Model file for the job. Use its own axes, mm. A direction names the side the tool comes from. Round coordinates to 2 decimals unless told otherwise and drop trailing zeros. Use a Markdown table: item, result. Add a question column.
Item 1: Tool access for faces 1 (the flat face through (-1, -304.8, 3)), 2 (the cylindrical face through (-219.67, -4.27, -106.67)): list every direction of +Z, -Z, +X, -X, +Y, -Y with a clear straight run to the whole face (end or side of a thin tool).
Item 2: Saw through at A-A on y = -169. Give the number of separate pieces and of enclosed holes in the cut face, then the cut area to 3 significant figures.
Item 3: Wall check: L1, parallel to X at y = -106, z = 20; L2, parallel to X at y = -13, z = -317; L3, parallel to X at y = 91, z = 204. Give the ranges that are in metal, low to high. Write a range as from..to.
Item 4: Two-plate mould, pull along X, no slides. Class faces 3 (the flat face through (3, -4, -228.6)), 4 (the cylindrical face through (-243.23, -4.09, 8.38)), 5 (the cylindrical face through (243.23, -4.09, -8.38)), 6 (the flat face through (4, -4, 584.2)): +X half, -X half, draft (parallel to the pull), parting line (faces both ways), or undercut.
Item 5: Pin check, flat tips, straight feed: P1, Ø10, axis at y = -227, z = -224, coming from the -X side; P2, Ø2, axis at y = -164.5, z = -183, coming from the -X side; P3, Ø1, axis at y = 111, z = -388.5, coming from the -X side. Stop position of each tip, or through.
```python
from build123d import *

# Parameters (mm, degrees)
F1_DEPTH = 304.8
F2_R     = 12.7
F4_DEPTH = 609.601


with BuildPart() as f1:
    # F0 (on Front) → F1 (new body, symmetric)
    with BuildSketch(Plane.XZ):
        with BuildLine():
            Line((304.8, 609.6), (-304.8, 609.6))
            ThreePointArc((-304.8, 609.6), (-243.217894, 0), (-304.8, -609.6))
            Line((-304.8, -609.6), (304.8, -609.6))
            ThreePointArc((304.8, -609.6), (243.217894, 0), (304.8, 609.6))
        make_face()
    extrude(amount=F1_DEPTH, both=True)

    # F2
    f2_edges = [f1.edges().sort_by_distance(p)[0] for p in [
        (304.8, 0, 609.6),
        (0, -304.8, 609.6),
        (-304.8, 0, 609.6),
        (0, 304.8, 609.6),
        (0, -304.8, -609.6),
        (304.8, 0, -609.6),
        (0, 304.8, -609.6),
        (-304.8, 0, -609.6),
        (243.217894, -304.8, 0),
        (-243.217894, -304.8, 0),
        (243.217894, 304.8, 0),
        (-243.217894, 304.8, 0),
    ]]
    fillet(f2_edges, radius=F2_R)

    # F3 (on face) → F4 (cut, through all)
    with BuildSketch(Plane.XZ.offset(304.8)):
        with BuildLine():
            ThreePointArc((248.302135, 431.8), (260.119024, 508.160601), (273.851838, 584.2))
            Line((273.851838, 584.2), (-273.851838, 584.2))
            ThreePointArc((-273.851838, 584.2), (-260.119024, 508.160601), (-248.302135, 431.8))
            Line((-248.302135, 431.8), (248.302135, 431.8))
        make_face()
        with BuildLine():
            ThreePointArc((273.851838, -584.2), (260.119024, -508.160601), (248.302135, -431.8))
            Line((248.302135, -431.8), (-248.302135, -431.8))
            ThreePointArc((-248.302135, -431.8), (-260.119024, -508.160601), (-273.851838, -584.2))
            Line((-273.851838, -584.2), (273.851838, -584.2))
        make_face()
        with BuildLine():
            ThreePointArc((244.805808, -406.4), (234.275634, -317.634344), (226.331339, -228.6))
            Line((226.331339, -228.6), (-226.331339, -228.6))
            ThreePointArc((-226.331339, -228.6), (-234.275634, -317.634344), (-244.805808, -406.4))
            Line((-244.805808, -406.4), (244.805808, -406.4))
        make_face()
        with BuildLine():
            ThreePointArc((224.542607, -203.2), (219.716122, -108.001944), (217.844134, -12.7))
            Line((217.844134, -12.7), (-217.844134, -12.7))
            ThreePointArc((-217.844134, -12.7), (-219.716122, -108.001944), (-224.542607, -203.2))
            Line((-224.542607, -203.2), (224.542607, -203.2))
        make_face()
        with BuildLine():
            ThreePointArc((217.844134, 12.7), (219.716122, 108.001944), (224.542607, 203.2))
            Line((224.542607, 203.2), (-224.542607, 203.2))
            ThreePointArc((-224.542607, 203.2), (-219.716122, 108.001944), (-217.844134, 12.7))
            Line((-217.844134, 12.7), (217.844134, 12.7))
        make_face()
        with BuildLine():
            ThreePointArc((226.331339, 228.6), (234.275634, 317.634344), (244.805808, 406.4))
            Line((244.805808, 406.4), (-244.805808, 406.4))
            ThreePointArc((-244.805808, 406.4), (-234.275634, 317.634344), (-226.331339, 228.6))
            Line((-226.331339, 228.6), (226.331339, 228.6))
        make_face()
    extrude(amount=-F4_DEPTH, mode=Mode.SUBTRACT)


solid = f1.part
```
Entries:
| question | item | result |
|---|---|---|
| 1 | face 1 | +Z, -Z, +X, -X, -Y |
| 1 | face 2 | +Y, -Y |
| 2 | separate pieces | 1 |
| 2 | enclosed holes | 6 |
| 2 | area | 149,000 mm2 |
| 3 | L1 | -243.28..-217.88, 217.88..243.28 |
| 3 | L2 | -259.75..-234.21, 234.21..259.75 |
| 3 | L3 | -250.05..250.05 |
| 4 | face 3 | undercut |
| 4 | face 4 | -X half |
| 4 | face 5 | +X half |
| 4 | face 6 | undercut |
| 5 | P1 | x = -251.83 |
| 5 | P2 | x = -248.78 |
| 5 | P3 | x = -268.14 |
